Answer from the drawing. Dimensions are ordinates in mm from the lowest x, y and z of the part. A direction names the side the tool comes from. Give positions to 0.01 mm unless a question says otherwise; leave off trailing zeros. Loops run counter-clockwise (first coordinate to the right, second up) from the corner with the lowest first, then second, coordinate; pieces in that order, holes last. Notation, with made-up numbers: M 49.25,61 L 95.25,61 A22 ccw 95.25,86 Z; hole C 58.5,-7.5 d2. An arc over 180 degrees is marked long. Return JSON: item names as keys, results as strings. Group by question number.
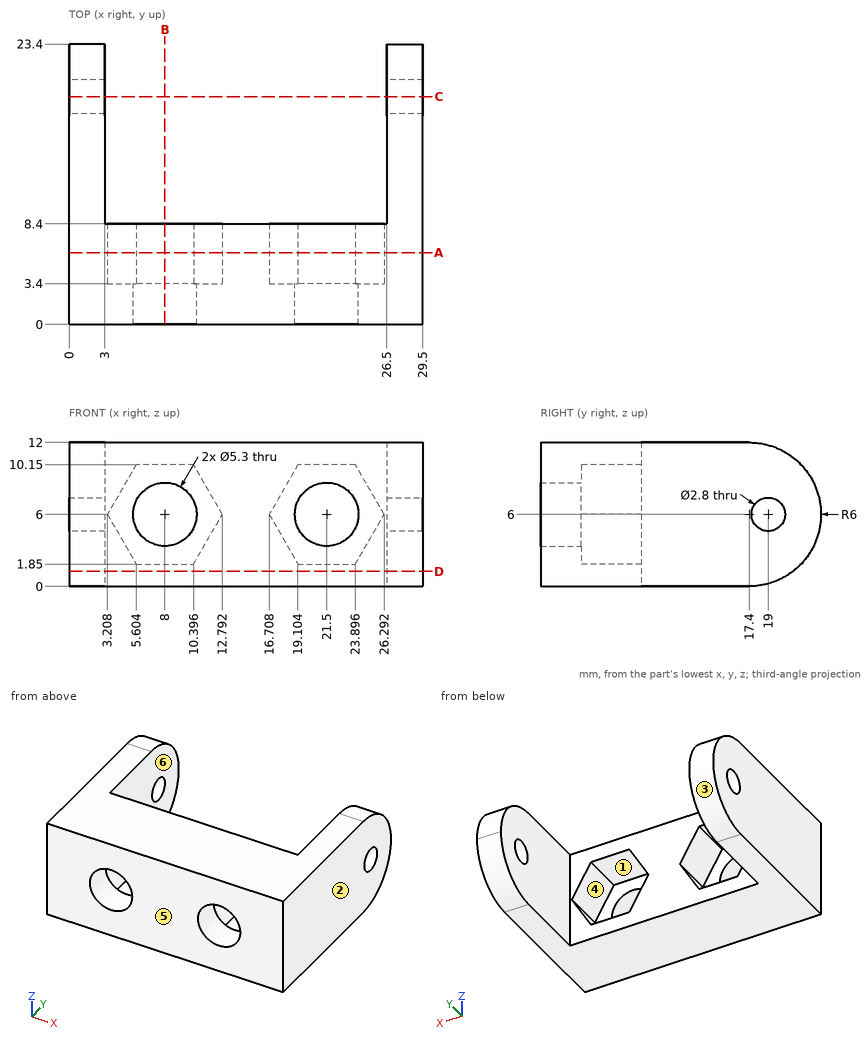
1. Find section B-B (x = 8). Write down the section's boundary in (y, z), and give its area (3 significant figures).
2. Straight lines are drawn through the part: line 1 along X through (y, z) = (9.75, 11.25); line 2 along Y through (x, z) = (2.15, 6); line 3 along X through (y, z) = (6, 2.5). For each, find the intervals that lie inside material, in ascending order.
3. Flat-ended cylindrical pins translate along their axes: P1, Ø1, axis at x = 19, z = 10.5, coming from the +Y side; P2, Ø4, axis at x = 23, z = 5, coming from the +Y side; P3, Ø1.7, axis at y = 19, z = 6, coming from the +X side. Find the tip coordinate at first contact, or state that the pin passes through.
4. The mould has two halves that part along X. Classify the marked faces 1, 2 and 3: +X half, -X half, draft (parallel to the pull), parting line (faces both ways), or undercut.
5. Find section A-A (y = 6). Write down the section's boundary in (x, z).
6. For the marked faces 4, 5 and 6, determine the directions among +Z, -Z, +X, -X, +Y, -Y from which every point of the face is accessible in a straight line to the end or side of a thin tool.
7. Find section D-D (z = 1.25). Write down the section's boundary in (x, y), and give its area (3 significant figures).
8. Find section C-C (y = 19). Write down the section's boundary in (x, z).
Result:
{
 "1": {"outline": "M 0,0 L 8.4,0 L 8.4,1.85 L 3.4,1.85 L 3.4,3.35 L 0,3.35 Z; M 0,8.65 L 3.4,8.65 L 3.4,10.15 L 8.4,10.15 L 8.4,12 L 0,12 Z", "area": "41.3 mm2"},
 "2": {"line 1": "x = 0 to 3, 26.5 to 29.5", "line 2": "y = 0 to 17.6, 20.4 to 23.4", "line 3": "x = 0 to 5.23, 10.77 to 18.73, 24.27 to 29.5"},
 "3": {"P1": "stops at y = 8.4", "P2": "stops at y = 3.4", "P3": "passes through"},
 "4": {"face 1": "undercut", "face 2": "+X half", "face 3": "draft"},
 "5": {"outline": "M 0,0 L 29.5,0 L 29.5,12 L 0,12 Z; hole M 3.21,6 L 5.6,1.85 L 10.4,1.85 L 12.79,6 L 10.4,10.15 L 5.6,10.15 Z; hole M 16.71,6 L 19.1,1.85 L 23.9,1.85 L 26.29,6 L 23.9,10.15 L 19.1,10.15 Z"},
 "6": {"face 4": "+Y", "face 5": "+Z, -Z, +X, -X, -Y", "face 6": "+Z, -Z, +Y"},
 "7": {"outline": "M 0,0 L 29.5,0 L 29.5,21.07 L 26.5,21.07 L 26.5,8.4 L 3,8.4 L 3,21.07 L 0,21.07 Z", "area": "324 mm2"},
 "8": {"outline": "M 0,0.22 L 3,0.22 L 3,4.6 L 0,4.6 Z; M 0,7.4 L 3,7.4 L 3,11.78 L 0,11.78 Z; M 26.5,0.22 L 29.5,0.22 L 29.5,4.6 L 26.5,4.6 Z; M 26.5,7.4 L 29.5,7.4 L 29.5,11.78 L 26.5,11.78 Z"}
}
